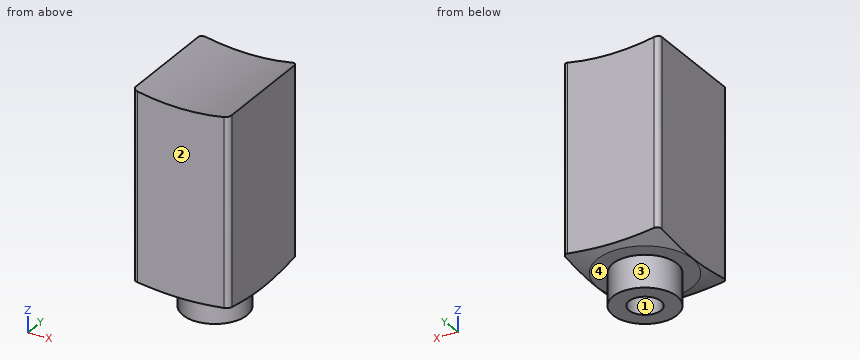
```python
from build123d import *

# Parameters (mm, degrees)
EXTRUSION1_DEPTH        = 12
ENL_V_MAT_EXTRU_1_DEPTH = 6
ESQUISSE3_R             = 2
ESQUISSE3_R_2           = 1
EXTRUSION2_DEPTH        = 2


with BuildPart() as part:
    # Esquisse1 → Extrusion1 (new body)
    with BuildSketch(Plane.XY):
        with BuildLine():
            Line((-2.7, 3.5), (2.7, 3.5))
            ThreePointArc((2.7, 3.5), (2.912132034, 3.412132034), (3, 3.2))
            Line((3, 3.2), (3, -3.2))
            ThreePointArc((3, -3.2), (2.912132034, -3.412132034), (2.7, -3.5))
            Line((2.7, -3.5), (-2.7, -3.5))
            ThreePointArc((-2.7, -3.5), (-2.912132034, -3.412132034), (-3, -3.2))
            Line((-3, -3.2), (-3, 3.2))
            ThreePointArc((-3, 3.2), (-2.912132034, 3.412132034), (-2.7, 3.5))
        make_face()
    extrude(amount=EXTRUSION1_DEPTH)

    # Esquisse2 → Enlèv. mat.-Extru.1 (cut, symmetric)
    with BuildSketch(Plane(origin=(0, 0, 0), x_dir=(1, 0, 0), z_dir=(0, 1, 0))):
        with BuildLine():
            Line((14, -25.674794331), (-14, -25.674794331))
            ThreePointArc((-14, -25.674794331), (0, -11.674794331), (14, -25.674794331))
        make_face()
    extrude(amount=ENL_V_MAT_EXTRU_1_DEPTH, both=True, mode=Mode.SUBTRACT)

    # Esquisse3 → Extrusion2 (add)
    with BuildSketch(Plane(origin=(0, 0, 0), x_dir=(-1, 0, 0), z_dir=(0, 0, -1))):
        with Locations(Location((0, 0, 0), (0, 0, 180))):
            Circle(ESQUISSE3_R)
        Circle(ESQUISSE3_R_2, mode=Mode.SUBTRACT)
    extrude(amount=EXTRUSION2_DEPTH)

    # Esquisse4 → Enlèvement de matière-Révolution1 (revolve, cut)
    with BuildSketch(Plane(origin=(0, 0, 0), x_dir=(1, 0, 0), z_dir=(0, 1, 0)), mode=Mode.PRIVATE) as enl_vement_de_mati_re_r_volution1_sk:
        Polygon((-5.932823797, -0.629669223), (-2.5, 0.1), (-2.5, 1.1), (-5.932823797, 1.1), align=None)
    revolve(enl_vement_de_mati_re_r_volution1_sk.sketch.rotate(Axis((0, 0, 13.123822536), (0, 0, -1)), 180), axis=Axis((0, 0, 13.123822536), (0, 0, -1)), mode=Mode.SUBTRACT)


solid = part.part
```
The listing builds one solid part. Answer for the finished solid, in the listing's coordinates (mm). Face numbers are marked on the shaded views. Coordinates: 2 decimals unless noted, no trailing zeros. Loops run counter-clockwise (first coordinate to the right, second up) from the corner with the lowest first, then second, coordinate; pieces in that order, holes last. Notation, with made-up numbers: M 0,48 L 59,48 A10 cw 59,56 Z; hole C -4.75,78.5 d8. An arc over 180 degrees is marked long. Answer as a JSON object with one key per item and string values. Group by question number.
Item 1: Section A-A (x = 0) is taken. Write down the section's boundary in (y, z).
Item 2: Determine the mould class of the marked faces 1, 2, 3 and 4 for opening direction Y: +Y half, -Y half, draft (parallel to the pull), parting line (faces both ways), or undercut.
Item 3: Each of these flat-tipped pins is pushed along its axis until it touches: P1, Ø1.6, axis at x = 0, y = 0, coming from the -Z side; P2, Ø2.5, axis at x = 0, y = 0, coming from the +Z side. Where does it stop, or does it pass through?
Item 4: Consider L1, parallel to Y at x = 0, z = -1.1; L2, parallel to Z at x = 0, y = 0.5; L3, parallel to Z at x = 1, y = -1.5. Determine where each line is inside the solid, lowest interval first.
Solved:
{
 "1": {"outline": "M -3.5,0.11 L -2.97,0 L -2,0 L -2,-2 L -1,-2 L -1,0 L 1,0 L 1,-2 L 2,-2 L 2,0 L 2.97,0 L 3.5,0.11 L 3.5,11.67 L -3.5,11.67 Z"},
 "2": {"face 1": "undercut", "face 2": "-Y half", "face 3": "parting line", "face 4": "draft"},
 "3": {"P1": "stops at z = 0", "P2": "stops at z = 11.73"},
 "4": {"L1": "y = -2 to -1, 1 to 2", "L2": "z = 0 to 11.67", "L3": "z = -2 to 11.71"}
}
